Can you work these out from the drawing? Everything is in mm from the part's minimum corner. Coordinates: 2 decimals unless noted, no trailing zeros. Loops run counter-clockwise (first coordinate to the right, second up) from the corner with the lowest first, then second, coordinate; pieces in that order, holes last. Notation, with made-up numbers: (16, 35.25) -> (63, 35.25) arc R29 ccw to (63, 57.25) -> close; hole circle Ø7 at (-1.75, 84.25). An arc over 180 degrees is marked (long way). Use one line per item in the form item = value. Start each with the question number.
(1) Imagine slicing it at C-C (z = 0.7). List the corners of the cut face in (x, y) for me.
(2) Imagine slicing it at D-D (x = 5). List the corners of the cut face in (y, z) for me, plus the area to 3 significant figures.
(3) I need wall thicknesses on line 1 (Y direction, x = 4, z = 0.8); line 2 (Y direction, x = 25.25, z = 0.15); line 3 (X direction, y = 14, z = 0.6). Which ranges of each line are inside material? Lowest first, please. Write a range as [from, to].
(4) Imagine slicing it at A-A (x = 15). List the corners of the cut face in (y, z) for me, plus the area to 3 significant figures.
(5) I'm going to push flat-ended pins straight in: pin 1 (12 mm diameter, centred on x = 4, y = 17, fed in from -Z); pin 2 (2.5 mm diameter, centred on x = 26, y = 26, fed in from +Z). Where does each tip first touch, or does it pass through?
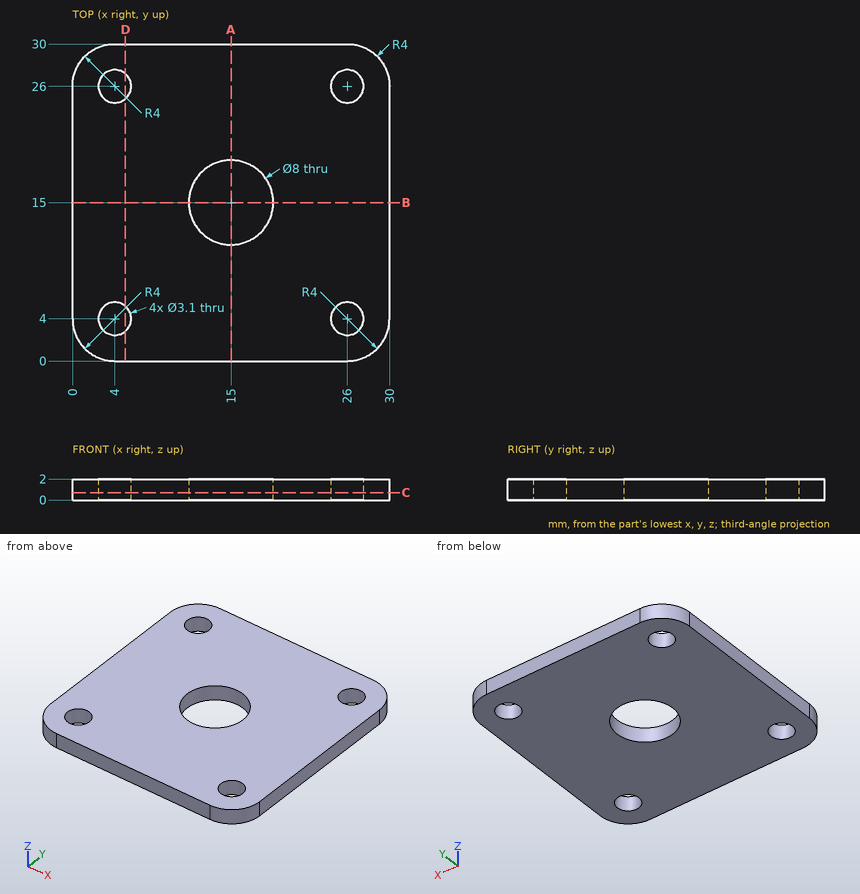
Worked out:
q1.outline = (0, 4) arc R4 ccw to (4, 0) -> (26, 0) arc R4 ccw to (30, 4) -> (30, 26) arc R4 ccw to (26, 30) -> (4, 30) arc R4 ccw to (0, 26) -> close; hole circle Ø3.1 at (4, 4); hole circle Ø3.1 at (4, 26); hole circle Ø8 at (15, 15); hole circle Ø3.1 at (26, 4); hole circle Ø3.1 at (26, 26)
q2.outline = (0, 0) -> (2.82, 0) -> (2.82, 2) -> (0, 2) -> close; (5.18, 0) -> (24.82, 0) -> (24.82, 2) -> (5.18, 2) -> close; (27.18, 0) -> (30, 0) -> (30, 2) -> (27.18, 2) -> close
q2.area = 50.5 mm2
q3.line_1 = [0, 2.45], [5.55, 24.45], [27.55, 30]
q3.line_2 = [0, 2.64], [5.36, 24.64], [27.36, 30]
q3.line_3 = [0, 11.13], [18.87, 30]
q4.outline = (0, 0) -> (11, 0) -> (11, 2) -> (0, 2) -> close; (19, 0) -> (30, 0) -> (30, 2) -> (19, 2) -> close
q4.area = 44.0 mm2
q5.pin_1 = 0
q5.pin_2 = through
